Verification items for the finished model (mm, model axes). A direction names the side the tool comes from. Coordinates: 2 decimals unless noted, no trailing zeros. Order: outer loops, then holes, each group sorted by start corner. A loop starts at its lowest first (then second) coordinate and runs counter-clockwise, first axis right, second up. Notation, with made-up numbers: (-11, -1) -> (39, -1) arc R24 ccw to (39, 25) -> close; hole circle Ø6 at (59.25, 68.25). An arc over 180 degrees is marked (long way). Write item = value, one per line. Start each with the question number.
1. Cross-section at B-B on z = 0. Record the cut outline in (x, y), plus the area to 3 significant figures.
2. Set-up check for faces 1 (the cylindrical face through (-18.916, -0.596, -2.685)), 2 (the flat face through (25, 0, 0)), 3 (the flat face through (13, -1, 3)): record each of +Z, -Z, +X, -X, +Y, -Y from which the full face is reachable in a straight line by a thin tool's end or side.
3. Cross-section at A-A on y = 0.5. Record the cut outline in (x, z), plus the area to 3 significant figures.
4. Cross-section at D-D on x = -16.5. Record the cut outline in (y, z), plus the area to 3 significant figures.
5. Go/stop test with flat-tipped pins: P1, Ø3, axis at x = -1.5, z = -3, coming from the -Y side; P2, Ø2, axis at y = -3, z = 2.5, coming from the +X side; P3, Ø3, axis at x = 13.5, z = -0.5, coming from the +Y side; P4, Ø2, axis at y = 2, z = 2.5, coming from the +X side. Record where each tip stops, or that it passes through.
6. Cross-section at C-C on x = 3. Record the cut outline in (y, z), plus the area to 3 significant figures.
7. Thickness scan on line 1 along X through (y, z) = (0, 2); line 2 along X through (y, z) = (0.75, 1.5); line 3 along Z through (x, y) = (-10.5, -3.5). Record the ranges inside material, lowest first. Write a range as from..to.
from build123d import *

# Parameters (mm, degrees)
F0_R          = 2.75
F1_DEPTH      = 25
F2_DEPTH      = 13
F3_R          = 2
F5_DEPTH      = 25
F5_DEPTH_BACK = 25
F7_R          = 0.5


with BuildPart() as f1:
    # F0 (on Right) → F1 (new body)
    with BuildSketch(Plane.YZ):
        Circle(F0_R)
    extrude(amount=F1_DEPTH)

    # F0 (on Right) → F2 (join)
    with BuildSketch(Plane.YZ):
        with BuildLine():
            ThreePointArc((0, -4), (2.8284271247, -2.8284271247), (4, 0))
            ThreePointArc((4, 0), (2.8284271247, 2.8284271247), (0, 4))
            ThreePointArc((0, 4), (-4, 0), (0, -4))
        make_face()
        Circle(F0_R, mode=Mode.SUBTRACT)
        with BuildLine():
            ThreePointArc((0, 4), (2.8284271247, 2.8284271247), (4, 0))
            ThreePointArc((4, 0), (2.8284271247, -2.8284271247), (0, -4))
            Line((0, -4), (5, -4))
            Line((5, -4), (5, 4))
            Line((5, 4), (0, 4))
        make_face()
    extrude(amount=F2_DEPTH)

    # F3
    f3_edges = [f1.edges().sort_by_distance(p)[0] for p in [
        (13, 5, 0),
    ]]
    fillet(f3_edges, radius=F3_R)

    # F4 (on Top) → F5 (cut, two sides)
    with BuildSketch(Plane.XY) as f5_sk:
        with BuildLine():
            Line((0, 1.9661990377), (0, -4.0338009623))
            Line((0, -4.0338009623), (10, -4.0338009623))
            ThreePointArc((10, -4.0338009623), (5.8309518948, 0.3511188625), (0, 1.9661990377))
        make_face()
    extrude(amount=F5_DEPTH, mode=Mode.SUBTRACT)
    extrude(f5_sk.sketch, amount=-F5_DEPTH_BACK, mode=Mode.SUBTRACT)

    # F6: F1 across face


with BuildPart() as f1_1:
    add(f1.part)
    add(f1.part.mirror(Plane(origin=(0, 3.4830995189, 0), x_dir=(0, -1, 0), z_dir=(-1, 0, 0))))

    # F7
    f7_edges = [f1_1.edges().sort_by_distance(p)[0] for p in [
        (13, -4, 0),
        (-13, -4, 0),
        (13, 1.5, -4),
        (13, 1.5, 4),
        (0, 5, 4),
        (12.414214, 4.414214, 4),
        (-13, 1.5, 4),
        (-12.414214, 4.414214, 4),
        (-12.414214, 4.414214, -4),
        (-13, 1.5, -4),
        (0, 5, -4),
        (12.414214, 4.414214, -4),
    ]]
    fillet(f7_edges, radius=F7_R)


solid = f1_1.part
Worked out:
q1.outline = (-25, -2.75) -> (-13, -2.75) -> (-13, -3.5) arc R0.5 ccw to (-12.5, -4) -> (-9.98, -4) arc R11.33 cw to (9.98, -4) -> (12.5, -4) arc R0.5 ccw to (13, -3.5) -> (13, -2.75) -> (25, -2.75) -> (25, 2.75) -> (13, 2.75) -> (13, 3) arc R2 ccw to (11, 5) -> (-11, 5) arc R2 ccw to (-13, 3) -> (-13, 2.75) -> (-25, 2.75) -> close
q1.area = 279 mm²
q2.face_1 = -X
q2.face_2 = +Z, -Z, +X, +Y, -Y
q2.face_3 = +X
q3.outline = (-25, -2.7) -> (-13, -2.7) -> (-13, -3.5) arc R0.5 ccw to (-12.5, -4) -> (-5.58, -4) -> (-5.58, 4) -> (-12.5, 4) arc R0.5 ccw to (-13, 3.5) -> (-13, 2.7) -> (-25, 2.7) -> close; (5.58, -4) -> (12.5, -4) arc R0.5 ccw to (13, -3.5) -> (13, -2.7) -> (25, -2.7) -> (25, 2.7) -> (13, 2.7) -> (13, 3.5) arc R0.5 ccw to (12.5, 4) -> (5.58, 4) -> close
q3.area = 248 mm²
q4.outline = circle Ø5.5 at (0, 0)
q4.area = 23.8 mm²
q5.P1 = 1.56
q5.P2 = 13
q5.P3 = 4.73
q5.P4 = 25
q6.outline = (1.56, -4) -> (4.5, -4) arc R0.5 ccw to (5, -3.5) -> (5, 3.5) arc R0.5 ccw to (4.5, 4) -> (1.56, 4) -> close
q6.area = 27.4 mm²
q7.line_1 = -25..-6.38, 6.38..25
q7.line_2 = -25..-5.11, 5.11..25
q7.line_3 = -1.94..1.94
